Study the drawing (mm; zero at the part's minimum x, y, z) and answer. A direction names the side the tool comes from. Coordinates: 2 decimals unless noted, no trailing zeros. Order: outer loops, then holes, each group sorted by start corner. A loop starts at its lowest first (then second) coordinate and runs counter-clockwise, first axis right, second up. Notation, with made-up numbers: (-23.5, 49) -> (32.5, 49) arc R17 cw to (32.5, 62) -> close; hole circle Ø7 at (2, 89). An arc over 180 degrees is marked (long way). One line per question, with ' | ' between items.
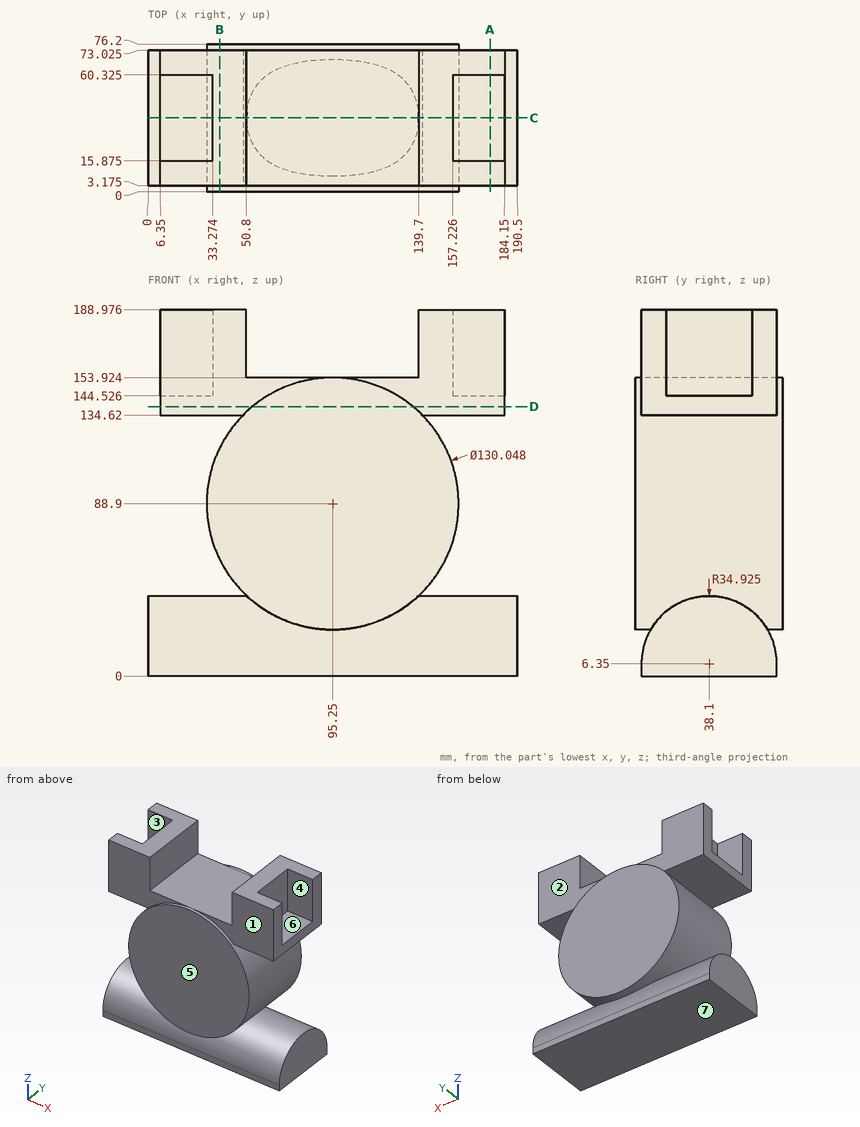
Item 1: Section C-C, the plane y = 38.1 is taken. Give the vertices of the cut face in (x, z) (3 decimals).
Computed values:
outline: (0, 0) -> (190.5, 0) -> (190.5, 41.275) -> (139.522, 41.275) arc R65.024 ccw to (141.486, 134.62) -> (184.15, 134.62) -> (184.15, 144.526) -> (157.226, 144.526) -> (157.226, 188.976) -> (139.7, 188.976) -> (139.7, 153.924) -> (50.8, 153.924) -> (50.8, 188.976) -> (33.274, 188.976) -> (33.274, 144.526) -> (6.35, 144.526) -> (6.35, 134.62) -> (49.014, 134.62) arc R65.024 ccw to (50.978, 41.275) -> (0, 41.275) -> close
Item 2: Section D-D, the plane z = 139 is taken. Give the vertices of the cut face in (x, y) (3 decimals), plus the area to 3 significant figures.
Computed values:
outline: (6.35, 3.175) -> (53.8, 3.175) -> (53.8, 0) -> (136.7, 0) -> (136.7, 3.175) -> (184.15, 3.175) -> (184.15, 73.025) -> (136.7, 73.025) -> (136.7, 76.2) -> (53.8, 76.2) -> (53.8, 73.025) -> (6.35, 73.025) -> close | area: 12,900 mm^2
Item 3: Determine the mould class of the marked faces 4, 5, 6 and 7 for opening direction Y: pulls with the +Y half, pulls with the -Y half, needs draft (parallel to the pull), parting line crosses it, or undercut.
Computed values:
face 4: undercut | face 5: pulls with the -Y half | face 6: undercut | face 7: needs draft
Item 4: Find the intervals of material crossed by L1, parallel to Z at x = 152, y = 37; L2, parallel to X at y = 50.5, z = 172; L3, parallel to Z at x = 48, y = 62.5, in increasing order.
Computed values:
L1: z = 0 to 41.26, 57.16 to 120.64, 134.62 to 188.98 | L2: x = 33.27 to 50.8, 139.7 to 157.23 | L3: z = 0 to 31.34, 44.23 to 133.57, 134.62 to 188.98
Item 5: Each of these flat-tipped pins is pushed along its axis until it touches: pin 1 Ø17.5 at (y, z) = (34.5, 175) entering from +X; pin 2 Ø3 at (y, z) = (44, 138) entering from +X; pin 3 Ø3 at (x, z) = (163, 148.5) entering from +Y (3 decimals); pin 4 Ø10 at (x, y) = (164.5, 51.5) entering from -Z. Where does it stop, or does it pass through?
Computed values:
pin 1: stops at x = 157.23 | pin 2: stops at x = 184.15 | pin 3: stops at y = 73.025 | pin 4: stops at z = 0
Item 6: Section B-B, the plane x = 37 is taken. Give the vertices of the cut face in (y, z) (3 decimals).
Computed values:
outline: (0, 60.003) -> (76.2, 60.003) -> (76.2, 117.797) -> (0, 117.797) -> close; (3.175, 0) -> (73.025, 0) -> (73.025, 6.35) arc R34.925 ccw to (3.175, 6.35) -> close; (3.175, 134.62) -> (73.025, 134.62) -> (73.025, 188.976) -> (3.175, 188.976) -> close
Item 7: Section A-A, the plane x = 176.5 is taken. Give the vertices of the cut face in (y, z) (3 decimals), plus the area to 3 significant figures.
Computed values:
outline: (3.175, 0) -> (73.025, 0) -> (73.025, 6.35) arc R34.925 ccw to (3.175, 6.35) -> close; (3.175, 134.62) -> (73.025, 134.62) -> (73.025, 188.976) -> (60.325, 188.976) -> (60.325, 144.526) -> (15.875, 144.526) -> (15.875, 188.976) -> (3.175, 188.976) -> close | area: 4,180 mm^2
Item 8: For the marked faces 1, 2 and 3, determine the directions among +Z, -Z, +X, -X, +Y, -Y from which every point of the face is accessible in a straight line to the end or side of a thin tool.
Computed values:
face 1: +Z, +X, -Y | face 2: +Z, +X, +Y | face 3: +Z, -X
